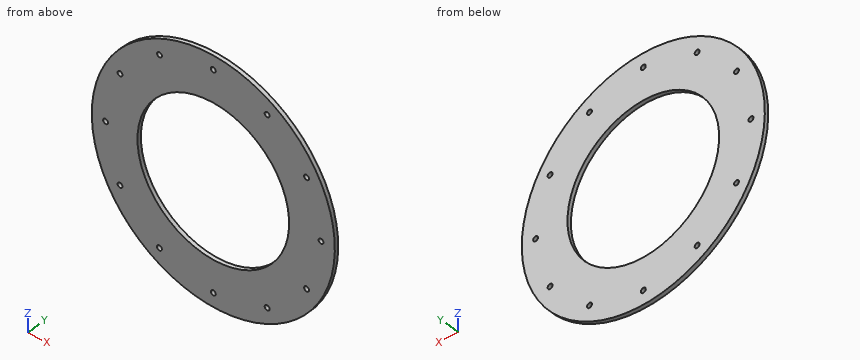
from build123d import *

# Parameters (mm, degrees)
SKETCH1_R           = 79
SKETCH1_R_2         = 49.3
BOSS_EXTRUDE1_DEPTH = 2.5
SKETCH2_R           = 1.6
CUT_EXTRUDE1_DEPTH  = 112.750838923


with BuildPart() as part:
    # Sketch1 → Boss-Extrude1 (new body)
    with BuildSketch(Plane(origin=(0, 0, 0), x_dir=(1, 0, 0), z_dir=(0, 1, 0))):
        with Locations(Location((0, 0, 0), (0, 0, 270))):
            Circle(SKETCH1_R)
        with Locations(Location((0, 0, 0), (0, 0, 270))):
            Circle(SKETCH1_R_2, mode=Mode.SUBTRACT)
    extrude(amount=BOSS_EXTRUDE1_DEPTH)

    # Sketch2 → Cut-Extrude1 (cut, through all)
    with BuildSketch(Plane(origin=(0, 2.5, 0), x_dir=(1, 0, 0), z_dir=(0, 1, 0))):
        with Locations(Location((0, 70, 0), (0, 0, 270))):
            Circle(SKETCH2_R)
        with Locations(Location((35, 60.621778265, 0), (0, 0, 270))):
            Circle(SKETCH2_R)
        with Locations(Location((60.621778265, 35, 0), (0, 0, 270))):
            Circle(SKETCH2_R)
        with Locations(Location((70, 0, 0), (0, 0, 270))):
            Circle(SKETCH2_R)
        with Locations(Location((60.621778265, -35, 0), (0, 0, 270))):
            Circle(SKETCH2_R)
        with Locations(Location((35, -60.621778265, 0), (0, 0, 270))):
            Circle(SKETCH2_R)
        with Locations(Location((0, -70, 0), (0, 0, 270))):
            Circle(SKETCH2_R)
        with Locations(Location((-35, -60.621778265, 0), (0, 0, 270))):
            Circle(SKETCH2_R)
        with Locations(Location((-60.621778265, -35, 0), (0, 0, 270))):
            Circle(SKETCH2_R)
        with Locations(Location((-70, 0, 0), (0, 0, 270))):
            Circle(SKETCH2_R)
        with Locations(Location((-60.621778265, 35, 0), (0, 0, 270))):
            Circle(SKETCH2_R)
        with Locations(Location((-35, 60.621778265, 0), (0, 0, 270))):
            Circle(SKETCH2_R)
    extrude(amount=-CUT_EXTRUDE1_DEPTH, mode=Mode.SUBTRACT)


solid = part.part
Verification items for the finished model (mm, model axes). Coordinates: 2 decimals unless noted, no trailing zeros. Order: outer loops, then holes, each group sorted by start corner. A loop starts at its lowest first (then second) coordinate and runs counter-clockwise, first axis right, second up.
Item 1: Section check A-A, the plane z = -47. Enter the section's corners in (x, y).
Filled in:
outline: (-63.5, 0) - (-14.88, 0) - (-14.88, 2.5) - (-63.5, 2.5) - close; (14.88, 0) - (63.5, 0) - (63.5, 2.5) - (14.88, 2.5) - close
Item 2: Section check C-C, the plane y = 0.6. Give the number of separate pieces and of enclosed holes in the cut face, then the cut area to 3 significant figures.
Filled in:
separate pieces: 1
enclosed holes: 13
area: 11,900 mm2
Item 3: Section check D-D, the plane z = -64.5. Enter the section's corners in (x, y), then the cut area to 3 significant figures.
Filled in:
outline: (-45.62, 0) - (45.62, 0) - (45.62, 2.5) - (-45.62, 2.5) - close
area: 228 mm2
Item 4: Material ranges on L1, parallel to X at y = 0.8, z = 0; L2, parallel to X at y = 1.55, z = -35; L3, parallel to Z at x = 70, y = 0.95, recorded low to high.
Filled in:
L1: x = -79 to -71.6, -68.4 to -49.3, 49.3 to 68.4, 71.6 to 79
L2: x = -70.82 to -62.22, -59.02 to -34.72, 34.72 to 59.02, 62.22 to 70.82
L3: z = -36.62 to -1.6, 1.6 to 36.62
Item 5: Section check B-B, the plane x = -18. Enter the section's corners in (y, z).
Filled in:
outline: (0, -76.92) - (2.5, -76.92) - (2.5, -45.9) - (0, -45.9) - close; (0, 45.9) - (2.5, 45.9) - (2.5, 76.92) - (0, 76.92) - close
